from build123d import *

# Parameters (mm, degrees)
F0_R     = 21.125
F2_R     = 21.575
F6_DEPTH = 5


with BuildPart() as f5:
    # F0 (on Top) → F5 section 0
    with BuildSketch(Plane.XY):
        Circle(F0_R)
    # F2 (on offset) → F5 section 1
    with BuildSketch(Plane.XY.offset(19)):
        Circle(F2_R)
    loft()

    # F4 (on offset) → F6 (join, through all)
    with BuildSketch(Plane.XY.offset(24)):
        Polygon((4.8545051575, 35.0056151581), (0.9513065061, 35.1146380116), (-2.9495599623, 35.0381506747), (-7.3858366721, 34.5027381994), (-11.4396800482, 33.431911015), (-14.6521593676, 32.4375728429), (-17.788150233, 30.9843078571), (-20.0827770418, 29.607532442), (-22.9128230274, 27.1599287256), (-24.6720395948, 25.1712512644), (-25.8193485314, 23.4885242679), (-26.9666664035, 21.4233594698), (-27.961007368, 19.1287304272), (-28.9760252346, 16.7291352786), (-29.7340651287, 14.6715869345), (-30.3550512956, 12.5905871947), (-30.8553268874, 10.1346778688), (-31.2450337726, 7.5703957518), (-31.3471315616, 4.5074330419), (-31.3471315616, 1.7507681666), (-31.2960826671, -0.9548455803), (-31.1429359836, -3.9157082674), (-30.8876915112, -6.3660775418), (-30.5813892087, -9.0716912887), (-30.0198513693, -11.8794072923), (-28.6502880738, -15.241816491), (-27.0111655274, -18.823602796), (-25.1899182536, -21.8590149189), (-22.3366308581, -24.8944315096), (-19.1798022503, -27.1406364806), (-15.2337664905, -29.2654249666), (-11.2270224883, -30.6010063007), (-7.7059444257, -31.4509216951), (-4.4884075754, -31.9365876348), (-0.7852047855, -32.1794206046), (2.4930403073, -32.1794206046), (5.7105771576, -31.9972958772), (9.3530806406, -31.5116299376), (12.6313257334, -30.8438392705), (16.820194463, -29.447549694), (20.8269295296, -27.3834694504), (23.8623461203, -24.7730150247), (26.7156335159, -21.7376029018), (28.9618384868, -18.155812129), (30.2974198209, -13.7241104295), (31.6937093974, -8.4424933357), (32.300791822, -3.585833939), (32.5436247918, 0.7244512755), (32.4328684384, 5.9111592441), (31.8553135951, 10.6038152433), (30.7723898868, 15.7296362581), (29.111915803, 20.3500951095), (26.3685180109, 24.6095816254), (23.3363405633, 28.3637048611), (18.643684564, 31.4680761057), (13.7344482909, 33.3451377235), (9.3305719472, 34.5002518779), align=None)
    extrude(amount=-F6_DEPTH)


solid = f5.part
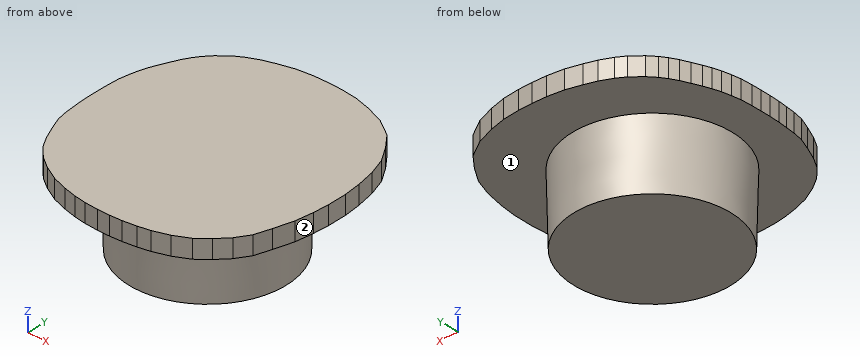
The listing builds one solid part. Answer for the finished solid, in the listing's coordinates (mm). Face numbers are marked on the shaded views. A direction names the side the tool comes from. Give positions to 0.01 mm unless a question says otherwise; leave off trailing zeros. Write each loop counter-clockwise with the first axis right and the second up, starting at its lowest first coordinate (ties: lowest second). Pieces come first, ordered by that corner, then holes.
Item 1: Which of the six approach directions +Z, -Z, +X, -X, +Y, -Y give full straight-line access (tool end or side, diameter ignored) to the marked faces 1 and 2?
Item 2: Flat-ended cylindrical pins translate along their axes: P1, Ø1.5, axis at x = 8.5, y = -22, coming from the -Z side; P2, Ø4, axis at y = 21, z = 4.5, coming from the -X side; P3, Ø4, axis at x = -16.5, z = 11.5, coming from the +Y side. Find the tip coordinate at first contact, or state that the pin passes through.
Item 3: Section A-A, the plane x = 0 is taken. Write down the section's boundary in (y, z) (3 decimals).
Item 4: Find the intervals of material crossed by line 1 along Z through (x, y) = (-9, -20); line 2 along X through (y, z) = (-0.5, 18.75); line 3 along Y through (x, z) = (11, 12.25), in increasing order.
Item 5: Section C-C, the plane z = 5.75 is taken. Write down the section's boundary in (x, y).
Item 6: Section B-B, the plane z = 12.5 is taken. Write down the section's boundary in (x, y), plus the area to 3 significant figures.
Completed:
1. face 1: -Z
1. face 2: +Z, -Z, +X, -Y
2. P1: stops at z = 19
2. P2: stops at x = -9.48
2. P3: stops at y = 15.74
3. outline: (-32.179, 19) - (-21.575, 19) - (-21.125, 0) - (21.125, 0) - (21.575, 19) - (35.096, 19) - (35.096, 24) - (-32.179, 24) - close
4. line 1: z = 19 to 24
4. line 2: x = -21.56 to 21.56
4. line 3: y = -18.37 to 18.37
5. outline: circle Ø42.52 at (0, 0)
6. outline: circle Ø42.84 at (0, 0)
6. area: 1,440 mm2
